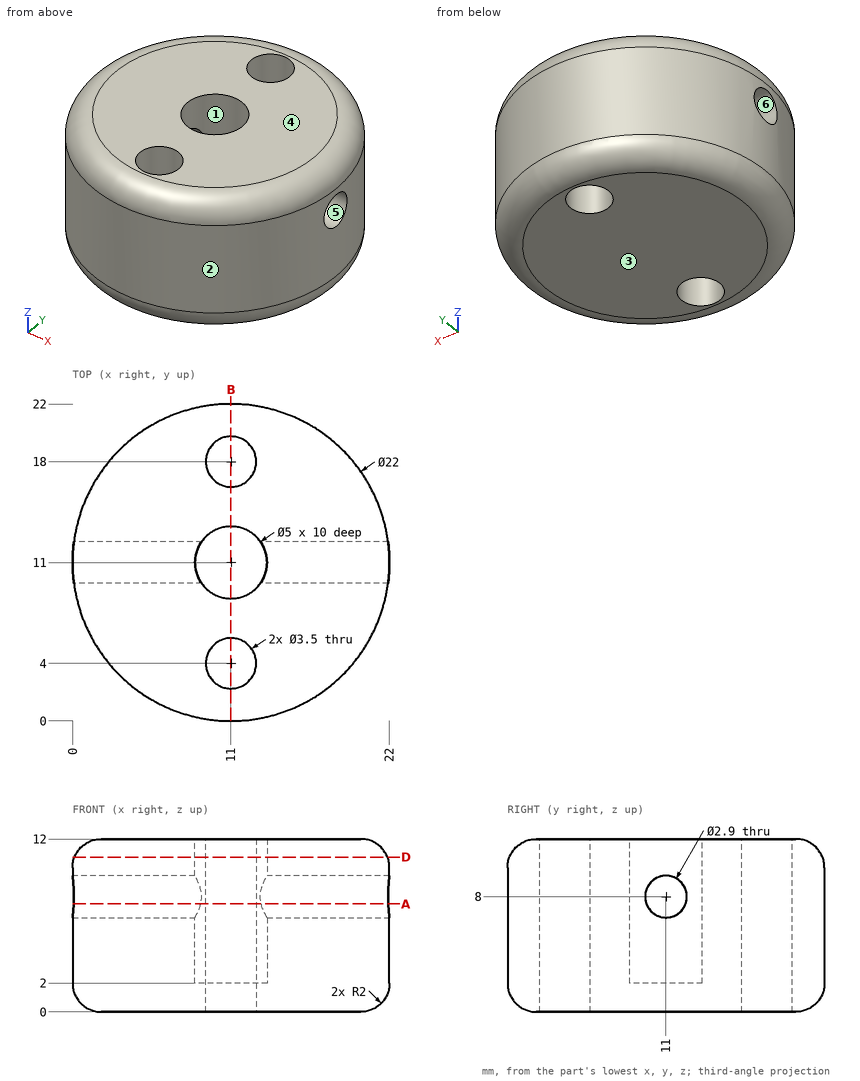
Drawing for the job (mm, zero at the part's lowest x, y, z). A direction names the side the tool comes from. Round coordinates to 2 decimals unless told otherwise and drop trailing zeros. Order: outer loops, then holes, each group sorted by start corner. A loop starts at its lowest first (then second) coordinate and runs counter-clockwise, first axis right, second up.
Item 1: Saw through at A-A on z = 7.5. Write the cut outline in (x, y), then the cut area to 3 significant figures.
Item 2: Pin check, flat tips, straight feed: pin 1 (3 mm diameter, centred on x = 11, y = 4, fed in from -Z); pin 2 (4 mm diameter, centred on x = 11, y = 11, fed in from +Z); pin 3 (3 mm diameter, centred on x = 14.5, z = 8, fed in from -Y); pin 4 (2 mm diameter, centred on y = 9, z = 4.5, fed in from +X). Stop position of each tip, or through.
Item 3: Probe line 1 along Y through (x, z) = (11, 8.25); line 2 along Y through (x, z) = (11.75, 9); line 3 along Y through (x, z) = (7.75, 7). List the from-to ranges inside material, lowest first.
Item 4: Tool access for the marked faces 1 and 2: list every direction of +Z, -Z, +X, -X, +Y, -Y with a clear straight run to the whole face (end or side of a thin tool).
Item 5: Saw through at B-B on x = 11. State how many separate pieces and enclosed holes the cut face has, then the cut area to 3 significant figures.
Item 6: Mould opens along Z. For the marked faces 3, 4, 5 and 6 say: pulls with the +Z half, pulls with the -Z half, needs draft (parallel to the pull), parting line crosses it, or undercut.
Item 7: Saw through at D-D on z = 10.75. Write the cut outline in (x, y).
Reported:
1. outline: (0.08, 9.64) arc R11 ccw to (21.92, 9.64) - (13.1, 9.64) arc R2.5 cw to (8.9, 9.64) - close; (0.08, 12.36) - (8.9, 12.36) arc R2.5 cw to (13.1, 12.36) - (21.92, 12.36) arc R11 ccw to start; hole circle Ø3.5 at (11, 4); hole circle Ø3.5 at (11, 18)
1. area: 294 mm2
2. pin 1: passes through
2. pin 2: stops at z = 2
2. pin 3: stops at y = 0.18
2. pin 4: stops at x = 21.95
3. line 1: y = 0 to 2.25, 5.75 to 8.5, 13.5 to 16.25, 19.75 to 22
3. line 2: y = 0.03 to 2.42, 5.58 to 8.62, 13.38 to 16.42, 19.58 to 21.97
3. line 3: y = 0.49 to 9.95, 12.05 to 21.51
4. face 1: +Z
4. face 2: +Z, -Z
5. separate pieces: 3
5. enclosed holes: 0
5. area: 127 mm2
6. face 3: pulls with the -Z half
6. face 4: pulls with the +Z half
6. face 5: undercut
6. face 6: undercut
7. outline: circle Ø21.71 at (11, 11); hole circle Ø5 at (11, 11); hole circle Ø3.5 at (11, 4); hole circle Ø3.5 at (11, 18)
